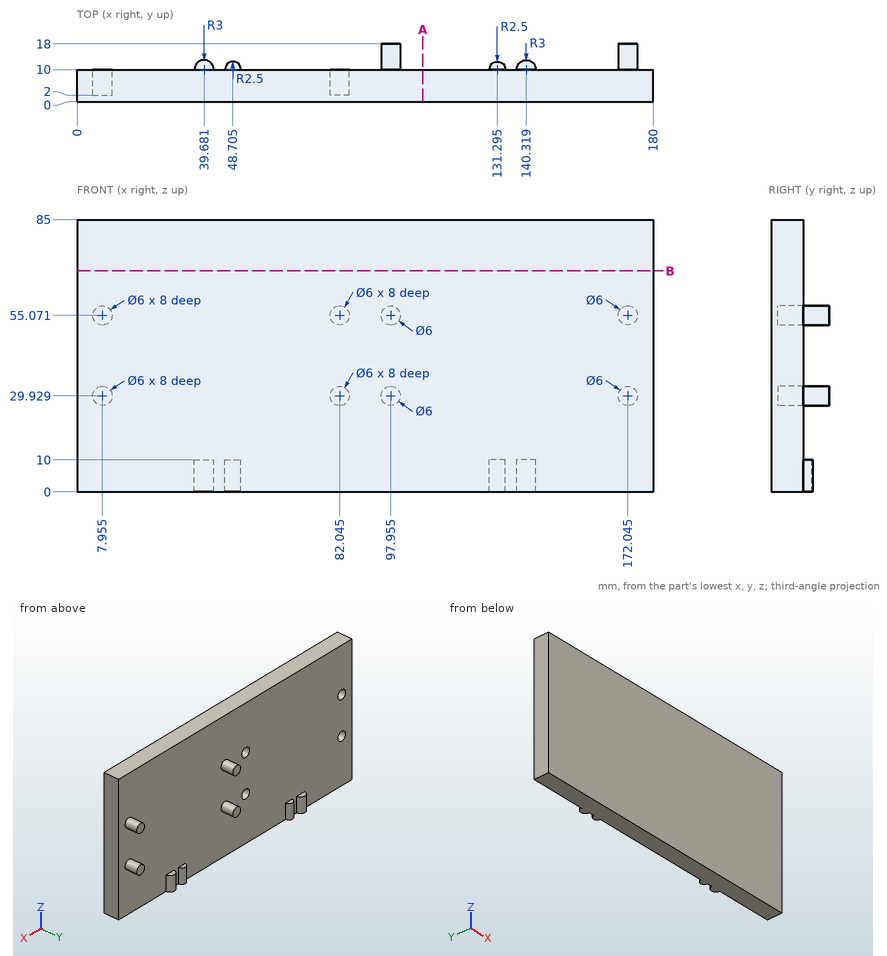
Input: dimensioned drawing with shaded views. Units: mm. Origin: part minimum x, y, z. Give positions to 0.01 mm unless a question says otherwise; leave off trailing zeros. Write each loop counter-clockwise with the first axis right and the second up, starting at its lowest first coordinate (ties: lowest second). Pieces come first, ordered by that corner, then holes. Notation, with made-up numbers: (32.25, 5) -> (73.25, 5) arc R11 ccw to (73.25, 20) -> close; hole circle Ø8 at (-17, 56). An arc over 180 degrees is marked (long way). Return JSON: item names as keys, results as strings. Group by question number.
1. Section A-A, the plane x = 108. Output: boundary loops of the cut face in (y, z), then the cut area to 3 significant figures.
2. Section B-B, the plane z = 69. Output: boundary loops of the cut face in (x, y), then the cut area to 3 significant figures.
3. Pin query (flat end, axial travel): pin 1 Ø6.5 at (x, z) = (9.5, 30.5) entering from +Y; pin 2 Ø5 at (x, z) = (7.95, 29.93) entering from +Y; pin 3 Ø0.9 at (x, y) = (140.5, 11) entering from +Z. Return the tip coordinate at first contact, or that it passes through.
4. Material intervals for line 1 (X direction, y = 6, z = 55.5) (1 decimal); line 2 (Y direction, x = 139, z = 45); line 3 (Z direction, x = 99.5, y = 13), sorted ascending. Write a range as from..to.
Determined:
{
 "1": {"outline": "(0, 0) -> (10, 0) -> (10, 85) -> (0, 85) -> close", "area": "850 mm2"},
 "2": {"outline": "(0, 0) -> (180, 0) -> (180, 10) -> (0, 10) -> close", "area": "1,800 mm2"},
 "3": {"pin 1": "stops at y = 10", "pin 2": "stops at y = 2", "pin 3": "stops at z = 10"},
 "4": {"line 1": "x = 0..5, 10.9..79.1, 85..180", "line 2": "y = 0..10", "line 3": "z = 27.36..32.5, 52.5..57.64"}
}
